Autodesk Inventor part; units mm, degrees
ref_plane "YZ Plane" through (0, 0, 0) normal (1, 0, 0) x (0, 1, 0)
ref_plane "XZ Plane" through (0, 0, 0) normal (0, 1, 0) x (-1, 0, 0)
ref_plane "XY Plane" through (0, 0, 0) normal (0, 0, 1) x (1, 0, 0)
sketch "スケッチ2" plane through (0, 0, 0) normal (0, 0, 1) x (1, 0, 0)
  line L0 (-31.5, 15) -> (31.5, 15)
  line L1 (31.5, 15) -> (31.5, -15)
  line L2 (31.5, -15) -> (-31.5, -15)
  line L3 (-31.5, -15) -> (-31.5, 15)
  line L4 (0, 21) -> (0, -21) construction
  line L5 (-44.1, 0) -> (44.1, 0) construction
  point P0 (0, 0)
  dimension "d1" = 63
  dimension "d2" = 30
  dimension "d3" = 15
  dimension "d4" = 31.5
extrude "押し出し1" add sketch "スケッチ2" along normal blind 3
sketch "スケッチ3" plane through (0, 0, 3) normal (0, 0, 1) x (1, 0, 0)
  line L0 (-31.5, -15) -> (31.5, -15) construction
  line L1 (31.5, -15) -> (31.5, 15) construction
  line L2 (31.5, 15) -> (-31.5, 15) construction
  line L3 (-31.5, 15) -> (-31.5, -15) construction
  line L4 (-44.1, 0) -> (44.1, 0) construction
  point P0 (0, 0)
  point P1 (-16.5, 0)
  point P2 (16.5, 0)
  dimension "d7" = 15
  dimension "d8" = 15
hole "穴1" at (-16.5, 0, 3) at (16.5, 0, 3) direction (0, 0, -1) diameter 6.6 end through all
fillet "フィレット1" radius 2 4 edges at (-31.5, 15, 1.5) (31.5, 15, 1.5) (31.5, -15, 1.5) (-31.5, -15, 1.5)
equation "\"d3\" = 0.5 * d2"
equation "\"d4\" = 0.5 * d1"
properties part number "rocker_bogie_mount"
Verification items for the finished model (mm, model axes). Round coordinates to 2 decimals unless told otherwise and drop trailing zeros. Order: outer loops, then holes, each group sorted by start corner. A loop starts at its lowest first (then second) coordinate and runs counter-clockwise, first axis right, second up. Notation, with made-up numbers: (-39, -22) - (-31, -22) arc R20 ccw to (-31, -18) - close; hole circle Ø4 at (40, -14). An arc over 180 degrees is marked (long way). Use CSV: the item, a comma, the result in double quotes. Start each with the question number.
1) Section check B-B, the plane x = -16.5. Record the cut outline in (y, z).
2) Mould release check, pull along X, two halves, no side actions. Record for faces 1 (the cylindrical face through (13.23, 0.43, 1.48)), 2 (the cylindrical face through (-30.9, 14.43, 1.52)), 3 (the flat face through (0, 15, 1)): +X half, -X half, draft (parallel to the pull), parting line (faces both ways), or undercut.
3) Section check A-A, the plane y = 0. Record the cut outline in (x, z), plus the area to 3 significant figures.
4) Section check D-D, the plane x = 14. Record the cut outline in (y, z), plus the area to 3 significant figures.
5) Section check C-C, the plane z = 1.9. Record the cut outline in (x, y), plus the area to 3 significant figures.
6) Thickness scan on L1, parallel to X at y = 0, z = 1.8; L2, parallel to X at y = 1, z = 0.8; L3, parallel to Y at x = -16.5, z = 1.4. Record the ranges inside material, lowest first.
Answers:
1,outline,"(-15, 0) - (-3.3, 0) - (-3.3, 3) - (-15, 3) - close; (3.3, 0) - (15, 0) - (15, 3) - (3.3, 3) - close"
2,face 1,"undercut"
2,face 2,"-X half"
2,face 3,"draft"
3,outline,"(-31.5, 0) - (-19.8, 0) - (-19.8, 3) - (-31.5, 3) - close; (-13.2, 0) - (13.2, 0) - (13.2, 3) - (-13.2, 3) - close; (19.8, 0) - (31.5, 0) - (31.5, 3) - (19.8, 3) - close"
3,area,"149 mm²"
4,outline,"(-15, 0) - (-2.15, 0) - (-2.15, 3) - (-15, 3) - close; (2.15, 0) - (15, 0) - (15, 3) - (2.15, 3) - close"
4,area,"77.1 mm²"
5,outline,"(-31.5, -13) arc R2 ccw to (-29.5, -15) - (29.5, -15) arc R2 ccw to (31.5, -13) - (31.5, 13) arc R2 ccw to (29.5, 15) - (-29.5, 15) arc R2 ccw to (-31.5, 13) - close; hole circle Ø6.6 at (-16.5, 0); hole circle Ø6.6 at (16.5, 0)"
5,area,"1,820 mm²"
6,L1,"x = -31.5 to -19.8, -13.2 to 13.2, 19.8 to 31.5"
6,L2,"x = -31.5 to -19.64, -13.36 to 13.36, 19.64 to 31.5"
6,L3,"y = -15 to -3.3, 3.3 to 15"
